CAD build for the part. Positions are in the model's coordinates, mm. A direction names the side the tool comes from. Coordinates: 2 decimals unless noted, no trailing zeros. Write each loop counter-clockwise with the first axis right and the second up, starting at its lowest first coordinate (ties: lowest second). Pieces come first, ordered by that corner, then holes. Notation, with made-up numbers: (6.25, 87) -> (63.25, 87) arc R20 cw to (63.25, 104) -> close; hole circle Ø4 at (55.5, 42). An arc over 180 degrees is marked (long way). Answer as CSV lines item,"result". Start each with the question number.
```python
from build123d import *

# Parameters (mm, degrees)
SKETCH1_R           = 17.25
BOSS_EXTRUDE1_DEPTH = 40
SKETCH2_R           = 18.5
BOSS_EXTRUDE2_DEPTH = 24.5
SKETCH3_R           = 6
BOSS_EXTRUDE3_DEPTH = 6
SKETCH4_R           = 3
BOSS_EXTRUDE4_DEPTH = 15
CUT_EXTRUDE1_START  = -12
CUT_EXTRUDE1_DEPTH  = 12
SKETCH7_R           = 1.25
CUT_EXTRUDE2_DEPTH  = 5


with BuildPart() as part:
    # Sketch1 → Boss-Extrude1 (new body)
    with BuildSketch(Plane.XY):
        Circle(SKETCH1_R)
    extrude(amount=BOSS_EXTRUDE1_DEPTH)

    # Sketch2 → Boss-Extrude2 (add)
    with BuildSketch(Plane.XY.offset(40)):
        Circle(SKETCH2_R)
    extrude(amount=BOSS_EXTRUDE2_DEPTH)

    # Sketch3 → Boss-Extrude3 (add)
    with BuildSketch(Plane.XY.offset(64.5)):
        with Locations((0, -7)):
            Circle(SKETCH3_R)
    extrude(amount=BOSS_EXTRUDE3_DEPTH)

    # Sketch4 → Boss-Extrude4 (add)
    with BuildSketch(Plane.XY.offset(70.5)):
        with Locations((0, -7)):
            Circle(SKETCH4_R)
    extrude(amount=BOSS_EXTRUDE4_DEPTH)

    # Sketch5 → Cut-Extrude1 (cut)
    with BuildSketch(Plane.XY.offset(85.5).offset(CUT_EXTRUDE1_START)):
        with BuildLine():
            Line((0, -4.5), (1.658312395, -4.5))
            ThreePointArc((1.658312395, -4.5), (0, -4), (-1.658312395, -4.5))
            Line((-1.658312395, -4.5), (0, -4.5))
        make_face()
    extrude(amount=CUT_EXTRUDE1_DEPTH, mode=Mode.SUBTRACT)

    # Sketch7 → Cut-Extrude2 (cut)
    with BuildSketch(Plane.XY.offset(64.5)):
        with Locations((-15.5, 1.1641e-05)):
            Circle(SKETCH7_R)
        with Locations((-7.75, 13.4234054)):
            Circle(SKETCH7_R)
        with Locations((7.75, 13.4234054)):
            Circle(SKETCH7_R)
        with Locations((15.5, 1.1641e-05)):
            Circle(SKETCH7_R)
        with Locations((7.75, -13.423382117)):
            Circle(SKETCH7_R)
        with Locations((-7.75, -13.423382117)):
            Circle(SKETCH7_R)
    extrude(amount=-CUT_EXTRUDE2_DEPTH, mode=Mode.SUBTRACT)


solid = part.part
```
1. Cut at B-B (z = 6.5). Give the cut face in (x, y).
2. Tool access for faces 1 (the face through (-4.01, -18.06, 52.08)), 2 (the face through (-17, -5, 40)), 3 (the face through (8, 13, 59.5)): list every direction of +Z, -Z, +X, -X, +Y, -Y with a clear straight run to the whole face (end or side of a thin tool).
3. Flat gauge pins, fed straight in: P1, Ø8, axis at x = 14.5, z = 65, coming from the -Y side; P2, Ø2, axis at x = 7.75, y = 13.42, coming from the +Z side; P3, Ø1, axis at x = -12.5, z = 49.5, coming from the +Y side; P4, Ø5, axis at x = -7, y = -13, coming from the -Z side. Where does each tip first touch, or does it go through?
4. Cut at C-C (y = -2.5). Give the cut face in (x, z).
5. Wall check: line 1 (Y direction, x = 7.75, z = 60.85); line 2 (Z direction, x = -11, y = 1); line 3 (Y direction, x = 15.5, z = 62.95). Give the ranges that are in metal, low to high.
6. Mould opens along X. For faces 4 (the face through (-16, 0, 59.5)), 5 (the face through (0, -4.5, 79)), 6 (the face through (16.453, 5.181, 19.72)), 7 (the face through (-8, 13, 59.5)) say: pulls with the +X half, pulls with the -X half, needs draft (parallel to the pull), parting line crosses it, or undercut.
7. Cut at A-A (x = 0). Give the cut face in (y, z).
8. Cut at D-D (y = 3). Give the cut face in (x, z).
Geometry check:
1,outline,"circle Ø34.5 at (0, 0)"
2,face 1,"+Z, -Z"
2,face 2,"-Z"
2,face 3,"+Z"
3,P1,"y = -15.21"
3,P2,"z = 59.5"
3,P3,"y = 14.08"
3,P4,"z = 0"
4,outline,"(-18.33, 40) -> (-17.07, 40) -> (-17.07, 0) -> (17.07, 0) -> (17.07, 40) -> (18.33, 40) -> (18.33, 64.5) -> (3.97, 64.5) -> (3.97, 70.5) -> (-3.97, 70.5) -> (-3.97, 64.5) -> (-18.33, 64.5) -> close"
5,line 1,"-16.8 to -14.67, -12.17 to 12.17, 14.67 to 16.8"
5,line 2,"0 to 64.5"
5,line 3,"-10.1 to -1.25, 1.25 to 10.1"
6,face 4,"undercut"
6,face 5,"needs draft"
6,face 6,"parting line crosses it"
6,face 7,"undercut"
7,outline,"(-18.5, 40) -> (-17.25, 40) -> (-17.25, 0) -> (17.25, 0) -> (17.25, 40) -> (18.5, 40) -> (18.5, 64.5) -> (-1, 64.5) -> (-1, 70.5) -> (-4, 70.5) -> (-4, 73.5) -> (-4.5, 73.5) -> (-4.5, 85.5) -> (-10, 85.5) -> (-10, 70.5) -> (-13, 70.5) -> (-13, 64.5) -> (-18.5, 64.5) -> close"
8,outline,"(-18.26, 40) -> (-16.99, 40) -> (-16.99, 0) -> (16.99, 0) -> (16.99, 40) -> (18.26, 40) -> (18.26, 64.5) -> (-18.26, 64.5) -> close"
